For this review, use the dimensioned drawing (mm, ordinates from the lowest corner) and the shaded views. A direction names the side the tool comes from. Round coordinates to 2 decimals unless told otherwise and drop trailing zeros. Write each loop counter-clockwise with the first axis right and the second up, starting at its lowest first coordinate (ties: lowest second). Pieces come first, ordered by that corner, then holes. Notation, with made-up numbers: (40.25, 64.25) -> (71.25, 64.25) arc R33 cw to (71.25, 99.25) -> close; hole circle Ø6 at (40, -15.5). An arc over 180 degrees is marked (long way). Write each question's results on one line, items separated by ' | '. Start each with the question number.
Item 1: Add section B-B (x = 22.5). State the section outline as (y, z) points, plus the area to 4 significant figures.
Item 2: Tool access review of the marked faces 1 and 2: name each direction out of +Z, -Z, +X, -X, +Y, -Y from which nothing blocks a thin tool from reaching the whole face with its end or side.
Item 3: To check wall thickness, follow line 1 along X through (y, z) = (23, 11); line 2 along Z through (x, y) = (15.5, 37); line 3 along X through (y, z) = (30, 7.25). State the ranges of each line that lie inside material, in increasing order.
Item 4: Add section A-A (y = 29). State the section outline as (x, z) points, plus the area to 3 significant figures.
Item 5: Add section C-C (z = 12.75). State the section outline as (x, y) points.
Item 6: The part is to be moulded in two halves that separate along X. For the marked faces 3 and 4, say which applies: +X half, -X half, draft (parallel to the pull), parting line (faces both ways), or undercut.
Item 7: Add section D-D (y = 36.5). State the section outline as (x, z) points, plus the area to 3 significant figures.
Item 8: Clearance check with flat-ended pins moving along their axes: pin 1 (2 mm diameter, centred on y = 11.5, z = 2, fed in from +X); pin 2 (4 mm diameter, centred on x = 24, y = 36, fed in from +Z); pin 3 (2 mm diameter, centred on x = 17, z = 9.5, fed in from +Y); pin 4 (12 mm diameter, centred on x = 18, y = 6, fed in from -Z). State where each tip first meets the part, or that it passes through.
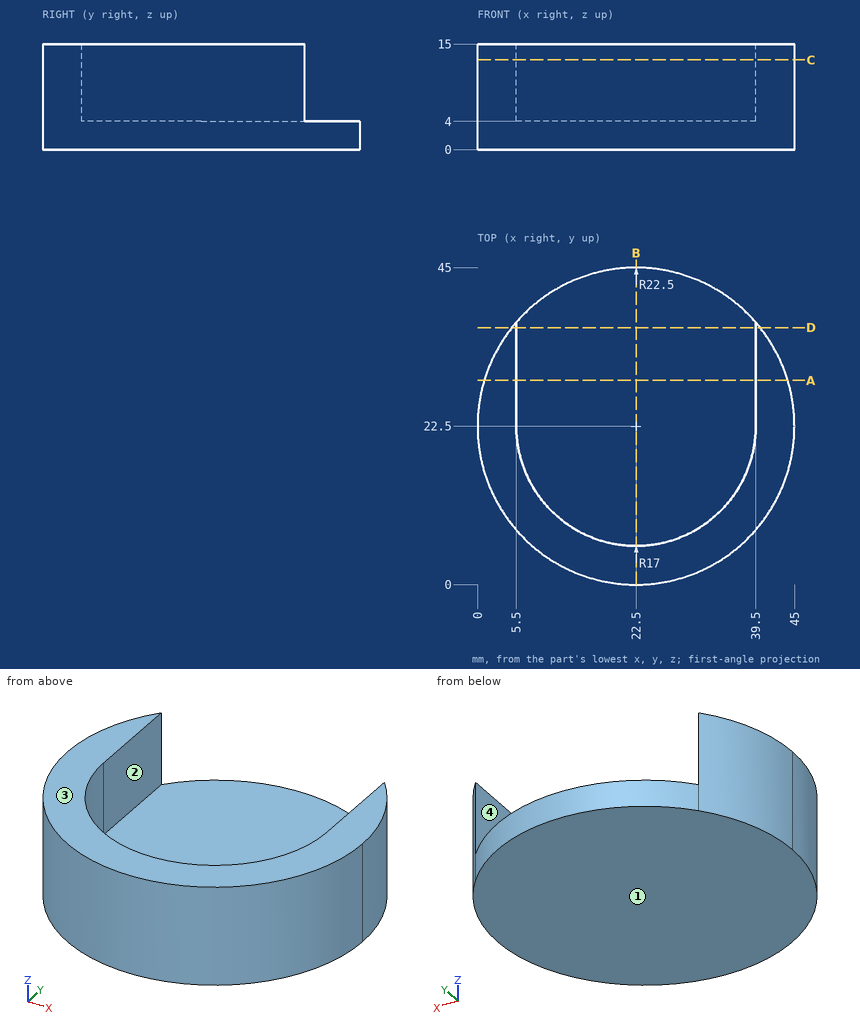
Responses:
1) outline: (0, 0) -> (45, 0) -> (45, 4) -> (5.5, 4) -> (5.5, 15) -> (0, 15) -> close | area: 240.5 mm^2
2) face 1: -Z, +X, -X, +Y, -Y | face 2: +Z, +Y
3) line 1: x = 0.01 to 5.5, 39.5 to 44.99 | line 2: z = 0 to 4 | line 3: x = 1.29 to 5.5, 39.5 to 43.71
4) outline: (0.96, 0) -> (44.04, 0) -> (44.04, 15) -> (39.5, 15) -> (39.5, 4) -> (5.5, 4) -> (5.5, 15) -> (0.96, 15) -> close | area: 272 mm^2
5) outline: (5.5, 22.5) -> (5.5, 37.24) arc R22.5 ccw (long way) to (39.5, 37.24) -> (39.5, 22.5) arc R17 cw to start
6) face 3: draft | face 4: undercut
7) outline: (4.89, 0) -> (40.11, 0) -> (40.11, 15) -> (39.5, 15) -> (39.5, 4) -> (5.5, 4) -> (5.5, 15) -> (4.89, 15) -> close | area: 154 mm^2
8) pin 1: stops at x = 42.66 | pin 2: stops at z = 4 | pin 3: stops at y = 6.79 | pin 4: stops at z = 0
